Autodesk Inventor part; units mm, degrees
ref_plane "YZ Plane" through (0, 0, 0) normal (1, 0, 0) x (0, 1, 0)
ref_plane "XZ Plane" through (0, 0, 0) normal (0, 1, 0) x (-1, 0, 0)
ref_plane "XY Plane" through (0, 0, 0) normal (0, 0, 1) x (1, 0, 0)
sketch "Sketch1" plane through (0, 0, 0) normal (0, 0, 1) x (1, 0, 0)
  line L0 (-75, 65) -> (75, 65)
  line L1 (75, 65) -> (75, -35)
  line L2 (75, -35) -> (-75, -35)
  line L3 (-75, -35) -> (-75, 65)
  point P0 (0, 0)
  dimension "d0" = 150
  dimension "d1" = 100
  dimension "d29" = 65
  dimension "d30" = 75
extrude "Extrusion1" add sketch "Sketch1" along normal blind 3.175
sketch "Sketch2" plane through (0, 0, 0) normal (0, 0, 1) x (1, 0, 0)
  line L0 (75, 65) -> (-75, 65)
  line L1 (-75, 65) -> (-75, -35)
  line L2 (75, -35) -> (75, 65)
  line L3 (-75, -35) -> (75, -35)
  point P0 (0, 0)
  point P1 (-70, 60)
  point P2 (70, 60)
  point P3 (70, -30)
  point P4 (-70, -30)
  dimension "d4" = 5
  dimension "d5" = 5
  dimension "d6" = 5
  dimension "d7" = 5
  dimension "d8" = 5
  dimension "d9" = 5
  dimension "d10" = 5
  dimension "d11" = 5
hole "Hole1" at (-70, 60, 0) at (70, 60, 0) at (70, -30, 0) at (-70, -30, 0) direction (0, 0, 1) diameter 3 end through all countersink diameter 4 countersink angle 90
fillet "Fillet1" radius 5 4 edges at (-75, 65, 1.5875) (75, 65, 1.5875) (75, -35, 1.5875) (-75, -35, 1.5875)
sketch "Sketch3" plane through (0, 0, 3.175) normal (0, 0, 1) x (1, 0, 0)
  circle A0 centre (0, 0) radius 3.25
  circle A1 centre (4.3841, -4.3841) radius 1.25
  circle A2 centre (-4.3841, 4.3841) radius 1.25
  dimension "d20" = 2.5
  dimension "d21" = 2.5
  dimension "d22" = 6.5
  dimension "d25" = 8.7681
  dimension "d26" = 8.7681
  dimension "d27" = 4.3841
  dimension "d28" = 4.3841
extrude "Extrusion2" cut sketch "Sketch3" against normal up to next
sketch "Sketch4" plane through (0, 0, 0) normal (0, 0, -1) x (-1, 0, 0)
  point P0 (0, 0)
  point P1 (-7.5, 13.5)
  point P2 (7.5, 13.5)
  point P3 (7.5, -15)
  point P4 (-7.5, -15)
  dimension "d33" = 15
  dimension "d34" = 15
  dimension "d35" = 13.5
  dimension "d36" = 15
  dimension "d37" = 7.5
  dimension "d38" = 15
  dimension "d39" = 7.5
  dimension "d40" = 13.5
hole "Hole2" at (7.5, 13.5, 0) at (-7.5, 13.5, 0) at (-7.5, -15, 0) at (7.5, -15, 0) direction (0, 0, 1) diameter 3 end through all countersink diameter 4 countersink angle 90
sketch "Sketch5" plane through (0, 0, 0) normal (0, 0, -1) x (-1, 0, 0)
  line L0 (70, 65) -> (-70, 65)
  line L1 (-75, 60) -> (-75, -30)
  line L2 (75, -30) -> (75, 60)
  point P0 (0, 0)
  point P1 (-20, 24)
  point P2 (-20, 31)
  point P3 (20, 31)
  point P4 (20, 24)
  dimension "d48" = 0
  dimension "d49" = 0
  dimension "d50" = 34
  dimension "d51" = 34
  dimension "d52" = 7
  dimension "d53" = 7
  dimension "d54" = 55
  dimension "d55" = 55
hole "Hole3" at (20, 24, 0) at (20, 31, 0) at (-20, 31, 0) at (-20, 24, 0) direction (0, 0, 1) diameter 3 end through all countersink diameter 4 countersink angle 90
properties part number "SheetPot"
Design review of the part built by this model. Coordinates are the model's own, in mm. Coordinates: 2 decimals unless noted, no trailing zeros. Order: outer loops, then holes, each group sorted by start corner. A loop starts at its lowest first (then second) coordinate and runs counter-clockwise, first axis right, second up. Notation, with made-up numbers: (-19.75, 13) -> (-3.75, 13) arc R35 cw to (-3.75, 46) -> close; hole circle Ø1 at (-30, 52). An arc over 180 degrees is marked (long way). One line per item, written item: value. Start each with the question number.
Q1. Insertion check: pin 1 Ø3.5 at (x, y) = (7.5, -15) entering from -Z. The pin has a flat end and moves straight along its axis. Give the tip position at first contact, or say it passes through.
Q2. For probe 1 along Y at (x, z) = (20, 1.2); probe 2 along Y at (x, z) = (70, 1.8); probe 3 along X at (y, z) = (31, 1.2), list the stretches that pass through material, from the lowest coordinate up.
Q3. Mouldability with a two-part tool opening along X and no side actions: class faces 1 (the cylindrical face through (73, -34, 2)), 2 (the cylindrical face through (69.93, -31.5, 1.86)), 3 (the flat face through (-1, 65, 2)) as pulls with the +X half, pulls with the -X half, needs draft (parallel to the pull), parting line crosses it, or undercut.
Q4. Take a section at A-A, the plane x = 7.5. State the section outline as (y, z) points (3 decimals), then the cut area to 3 significant figures.
Q5. Take a section at B-B, the plane y = -15. State the section outline as (x, z) points (3 decimals).
Q6. Take a section at C-C, the plane y = 0. State the section outline as (x, z) points (3 decimals).
Values follow:
1. pin 1: stops at z = 0.25
2. probe 1: y = -35 to 22.5, 25.5 to 29.5, 32.5 to 65
2. probe 2: y = -35 to -31.5, -28.5 to 58.5, 61.5 to 65
2. probe 3: x = -75 to -21.5, -18.5 to 18.5, 21.5 to 75
3. face 1: pulls with the +X half
3. face 2: undercut
3. face 3: needs draft
4. outline: (-35, 0) -> (-17, 0) -> (-16.5, 0.5) -> (-16.5, 3.175) -> (-35, 3.175) -> close; (-13.5, 0.5) -> (-13, 0) -> (11.5, 0) -> (12, 0.5) -> (12, 3.175) -> (-13.5, 3.175) -> close; (15, 0.5) -> (15.5, 0) -> (65, 0) -> (65, 3.175) -> (15, 3.175) -> close
4. area: 298 mm2
5. outline: (-75, 0) -> (-9.5, 0) -> (-9, 0.5) -> (-9, 3.175) -> (-75, 3.175) -> close; (-6, 0.5) -> (-5.5, 0) -> (5.5, 0) -> (6, 0.5) -> (6, 3.175) -> (-6, 3.175) -> close; (9, 0.5) -> (9.5, 0) -> (75, 0) -> (75, 3.175) -> (9, 3.175) -> close
6. outline: (-75, 0) -> (-3.25, 0) -> (-3.25, 3.175) -> (-75, 3.175) -> close; (3.25, 0) -> (75, 0) -> (75, 3.175) -> (3.25, 3.175) -> close
